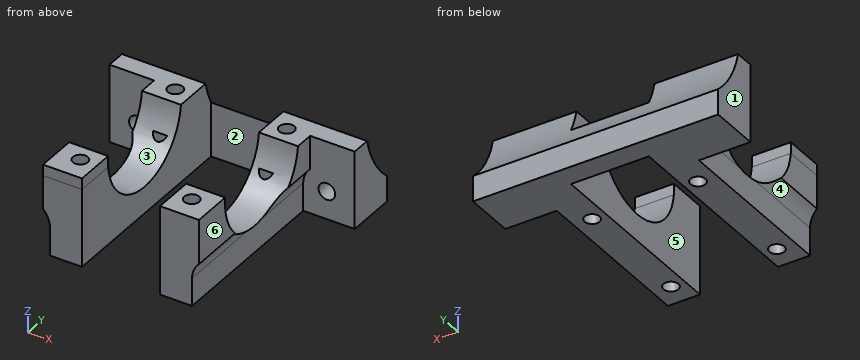
from build123d import *

# Parameters (mm, degrees)
F0_W      = 7
F0_H      = 31
F1_DEPTH  = 14
F2_R      = 1.35
F3_DEPTH  = 8
F4_R      = 10.2
F5_DEPTH  = 30
F6_R      = 1.35
F7_DEPTH  = 9
F8_R      = 1.5
F9_DEPTH  = 7
F10_R     = 18
F11_DEPTH = 44.001
F13_DEPTH = 31
F14_W     = 7
F14_H     = 7.299138
F14_R     = 1.35
F15_DEPTH = 2


with BuildPart() as f1:
    # F0 (on Top) → F1 (new body)
    with BuildSketch(Plane.XY):
        with Locations((-10.5, 15.5)):
            Rectangle(F0_W, F0_H)
        Polygon((-22, 31), (-14, 31), (-7, 31), (-7, 36), (7, 36), (7, 31), (14, 31), (22, 31), (22, 40), (-22, 40), align=None)
        with Locations((10.5, 15.5)):
            Rectangle(F0_W, F0_H)
    extrude(amount=F1_DEPTH)

    # F2 (on face) → F3 (cut)
    with BuildSketch(Plane.XY.offset(14)):
        with Locations((-10, 4.2)):
            Circle(F2_R)
        with Locations((-10, 30.7)):
            Circle(F2_R)
        with Locations((10, 30.7)):
            Circle(F2_R)
        with Locations((10, 4.2)):
            Circle(F2_R)
    extrude(amount=-F3_DEPTH, mode=Mode.SUBTRACT)

    # F4 (on face) → F5 (cut)
    with BuildSketch(Plane(origin=(-14, 0, 0), x_dir=(0, -1, 0), z_dir=(-1, 0, 0))):
        with Locations((-17.45, 15)):
            Circle(F4_R)
    extrude(amount=-F5_DEPTH, mode=Mode.SUBTRACT)

    # F6 (on face) → F7 (cut)
    with BuildSketch(Plane(origin=(0, 0, 0), x_dir=(1, 0, 0), z_dir=(0, 0, -1))):
        with Locations((9.5, -4.2)):
            Circle(F6_R)
        with Locations((-9.5, -4.2)):
            Circle(F6_R)
        with Locations((9.5, -26.2)):
            Circle(F6_R)
        with Locations((-9.5, -26.2)):
            Circle(F6_R)
    extrude(amount=-F7_DEPTH, mode=Mode.SUBTRACT)

    # F8 (on face) → F9 (cut)
    with BuildSketch(Plane.XZ.offset(-31)):
        with Locations((-17, 5)):
            Circle(F8_R)
        with Locations((17, 5)):
            Circle(F8_R)
    extrude(amount=-F9_DEPTH, mode=Mode.SUBTRACT)

    # F10 (on face) → F11 (cut, through all)
    with BuildSketch(Plane.YZ.offset(22)):
        with Locations((52, 18)):
            Circle(F10_R)
    extrude(amount=-F11_DEPTH, mode=Mode.SUBTRACT)

    # F12 (on face) → F13 (cut, through all)
    with BuildSketch(Plane.XZ):
        with BuildLine():
            Line((-12.75, -4.045816), (-12.75, 5))
            ThreePointArc((-12.75, 5), (-18.807251, 8.846602), (-19.712986, 1.728577))
            Line((-19.712986, 1.728577), (-12.75, -4.045816))
        make_face()
        with BuildLine():
            Line((12.75, -4.045816), (19.712986, 1.728577))
            ThreePointArc((19.712986, 1.728577), (18.807251, 8.846602), (12.75, 5))
            Line((12.75, 5), (12.75, -4.045816))
        make_face()
    extrude(amount=-F13_DEPTH, mode=Mode.SUBTRACT)

    # F14 (on face) → F15 (join)
    with BuildSketch(Plane.XY.offset(14)):
        with Locations((10.5, 3.649569)):
            Rectangle(F14_W, F14_H)
        with Locations((10, 4.2)):
            Circle(F14_R, mode=Mode.SUBTRACT)
        with Locations((-10.5, 3.649569)):
            Rectangle(F14_W, F14_H)
        with Locations((-10, 4.2)):
            Circle(F14_R, mode=Mode.SUBTRACT)
    extrude(amount=F15_DEPTH)


solid = f1.part
Check sheet for the modelled part. Datum: model origin and axes. Units: mm. Face numbers are marked on the shaded views. A direction names the side the tool comes from. Round coordinates to 2 decimals unless told otherwise and drop trailing zeros. Write each loop counter-clockwise with the first axis right and the second up, starting at its lowest first coordinate (ties: lowest second). Pieces come first, ordered by that corner, then holes. Notation, with made-up numbers: (85, -13) - (94, -13) arc R34 cw to (94, 17) - close; hole circle Ø9 at (-5, 38). An arc over 180 degrees is marked (long way). Return JSON: item names as keys, results as strings.
Q1. Draft check along Y on the marked faces 1, 2 and 3. Enter one of: released by +Y, released by -Y, zero draft, split by the parting line, or undercut.
Returned:
{"face 1": "zero draft", "face 2": "released by -Y", "face 3": "undercut"}
Q2. Access from +Z, -Z, +X, -X, +Y, -Y to the whole of each face (thin tool, end or side, straight path). Record for the marked faces 4, 5 and 6.
Returned:
{"face 4": "-Z, -X, -Y", "face 5": "+Z, -Z, -Y", "face 6": "+Z, -Z, +X, -Y"}
Q3. Cross-section at B-B (z = 13.5). Record the boundary of the cut face in (x, y), then the cut area to 3 significant figures.
Returned:
{"outline": "(-22, 31) - (-14, 31) - (-14, 27.54) - (-7, 27.54) - (-7, 34.57) - (-22, 34.57) - close; (-14, 0) - (-7, 0) - (-7, 7.36) - (-14, 7.36) - close; (7, 0) - (14, 0) - (14, 7.36) - (7, 7.36) - close; (7, 27.54) - (14, 27.54) - (14, 31) - (22, 31) - (22, 34.57) - (7, 34.57) - close; hole circle Ø2.7 at (-10, 4.2); hole circle Ø2.7 at (-10, 30.7); hole circle Ø2.7 at (10, 4.2); hole circle Ø2.7 at (10, 30.7)", "area": "236 mm²"}
Q4. Depth check by flat-ended pin: P1, Ø12, axis at x = -4, y = 23, coming from the +Z side; P2, Ø4.5, axis at x = -10, y = 4.2, coming from the -Z side; P3, Ø3.5, axis at x = -17, z = 5, coming from the -Y side; P4, Ø1, axis at y = 8.5, z = 7, coming from the -X side. Enter the tip coordinate at first touch or a pass-through.
Returned:
{"P1": "stops at z = 14", "P2": "stops at z = 0", "P3": "stops at y = 31", "P4": "stops at x = -13.56"}
Q5. Cross-section at A-A (z = 2.75). Record the boundary of the cut face in (x, y), then the cut area to 3 significant figures.
Returned:
{"outline": "(-22, 31) - (-12.75, 31) - (-12.75, 0) - (-7, 0) - (-7, 36) - (7, 36) - (7, 0) - (12.75, 0) - (12.75, 31) - (22, 31) - (22, 40) - (-22, 40) - close; hole circle Ø2.7 at (-9.5, 4.2); hole circle Ø2.7 at (-9.5, 26.2); hole circle Ø2.7 at (9.5, 4.2); hole circle Ø2.7 at (9.5, 26.2)", "area": "660 mm²"}
Q6. Cross-section at D-D (x = -17). Record the boundary of the cut face in (y, z).
Returned:
{"outline": "(31, 0) - (40, 0) - (40, 4.58) arc R18 cw to (34.45, 14) - (31, 14) - (31, 6.5) - (38, 6.5) - (38, 3.5) - (31, 3.5) - close"}
Q7. Scan lines: L1, parallel to X at y = 4.2, z = 4; L2, parallel to X at y = 8, z = 9. Record each from-to range of solid material in increasing order. Write a range as from..to.
Returned:
{"L1": "x = -12.75..-10.85, -8.15..-7, 7..8.15, 10.85..12.75", "L2": "x = -14..-7, 7..14"}
Q8. Cross-section at C-C (y = 26.2). Record the boundary of the cut face in (x, z), then the cut area to 3 significant figures.
Returned:
{"outline": "(-14, 8.01) arc R4.25 cw to (-12.75, 5) - (-12.75, 0) - (-10.85, 0) - (-10.85, 9) - (-8.15, 9) - (-8.15, 0) - (-7, 0) - (-7, 9.76) - (-14, 9.76) - close; (7, 0) - (8.15, 0) - (8.15, 9) - (10.85, 9) - (10.85, 0) - (12.75, 0) - (12.75, 5) arc R4.25 cw to (14, 8.01) - (14, 9.76) - (7, 9.76) - close", "area": "70.3 mm²"}
